Here's how the part is built. I have some questions about the finished solid (model axes, mm). Coordinates: 2 decimals unless noted, no trailing zeros. Loops run counter-clockwise (first coordinate to the right, second up) from the corner with the lowest first, then second, coordinate; pieces in that order, holes last. Notation, with made-up numbers: (-27.5, -9.75) -> (-0.5, -9.75) arc R8 ccw to (-0.5, 1.25) -> close; hole circle Ø5 at (5.5, -35). An arc over 180 degrees is marked (long way). Answer as a JSON object with one key per item and string values. Group by question number.
1) I want a section at A-A (y = 0). Write out the boundary of the cut face in (x, z).
2) I want a section at D-D (x = -15). Write out the boundary of the cut face in (y, z), then the cut area to 3 significant figures.
3) I want a section at C-C (z = 1.55). Write out the boundary of the cut face in (x, y), then the cut area to 3 significant figures.
4) If we mould it in two halves opening along X, with no side actions, what happens to faces 1 (the flat face through (6, 0, 2)), 2 (the cylindrical face through (-24.204, 18.559, 0.986)), 3 (the cylindrical face through (-16.586, 0.208, 0.986))? For each: +X half, -X half, draft (parallel to the pull), parting line (faces both ways), or undercut.
5) I need wall thicknesses on probe 1 along Y at (x, z) = (0, 0.75); probe 2 along X at (y, z) = (-1, 0.2); probe 3 along Y at (x, z) = (-15, 1.2). Which ranges of each line are inside material? Lowest first, please. Write a range as [from, to].
6) I want a section at B-B (x = 0). Write out the boundary of the cut face in (y, z).
Autodesk Inventor part; units mm, degrees
ref_plane "YZ Plane" through (0, 0, 0) normal (1, 0, 0) x (0, 1, 0)
ref_plane "XZ Plane" through (0, 0, 0) normal (0, 1, 0) x (-1, 0, 0)
ref_plane "XY Plane" through (0, 0, 0) normal (0, 0, 1) x (1, 0, 0)
sketch "スケッチ1" plane through (0, 0, 0) normal (0, 0, 1) x (1, 0, 0)
  circle A0 centre (0, 0) radius 30.5
  dimension "d0" = 61
extrude "押し出し1" add sketch "スケッチ1" along normal blind 2
sketch "スケッチ2" plane through (0, 0, 2) normal (0, 0, 1) x (1, 0, 0)
  circle A0 centre (0, 0) radius 4
  dimension "d3" = 8
extrude "押し出し2" cut sketch "スケッチ2" against normal blind 2
sketch "スケッチ3" plane through (0, 0, 2) normal (0, 0, 1) x (1, 0, 0)
  circle A0 centre (-15, 0) radius 1.6
  circle A1 centre (15, 0) radius 1.6
  point P0 (0, 0)
  dimension "d6" = 3.2
  dimension "d7" = 3.2
  dimension "d8" = 15
  dimension "d9" = 15
hole "穴1" at (-15, 0, 2) at (15, 0, 2) direction (0, 0, -1) diameter 3.2 depth 2
equation "\"BendRadius\" = Thickness"
equation "\"BendReliefWidth\" = Thickness"
equation "\"BendReliefDepth\" = 0.5 * Thickness"
equation "\"CornerReliefSize\" = 4 * Thickness"
equation "\"MinimumRemnant\" = 2 * Thickness"
equation "\"TransitionRadius\" = BendRadius"
equation "\"JacobiRadiusSize\" = BendRadius"
equation "\"GapSize\" = Thickness"
properties part number "nhk36"
Determined:
{
 "1": {"outline": "(-30.5, 0) -> (-16.6, 0) -> (-16.6, 2) -> (-30.5, 2) -> close; (-13.4, 0) -> (-4, 0) -> (-4, 2) -> (-13.4, 2) -> close; (4, 0) -> (13.4, 0) -> (13.4, 2) -> (4, 2) -> close; (16.6, 0) -> (30.5, 0) -> (30.5, 2) -> (16.6, 2) -> close"},
 "2": {"outline": "(-26.56, 0) -> (-1.6, 0) -> (-1.6, 2) -> (-26.56, 2) -> close; (1.6, 0) -> (26.56, 0) -> (26.56, 2) -> (1.6, 2) -> close", "area": "99.8 mm^2"},
 "3": {"outline": "circle Ø61 at (0, 0); hole circle Ø3.2 at (-15, 0); hole circle Ø8 at (0, 0); hole circle Ø3.2 at (15, 0)", "area": "2,860 mm^2"},
 "4": {"face 1": "draft", "face 2": "parting line", "face 3": "undercut"},
 "5": {"probe 1": "[-30.5, -4], [4, 30.5]", "probe 2": "[-30.48, -16.25], [-13.75, -3.87], [3.87, 13.75], [16.25, 30.48]", "probe 3": "[-26.56, -1.6], [1.6, 26.56]"},
 "6": {"outline": "(-30.5, 0) -> (-4, 0) -> (-4, 2) -> (-30.5, 2) -> close; (4, 0) -> (30.5, 0) -> (30.5, 2) -> (4, 2) -> close"}
}
